Verification items for the finished model (mm, model axes). A direction names the side the tool comes from. Coordinates: 2 decimals unless noted, no trailing zeros. Order: outer loops, then holes, each group sorted by start corner. A loop starts at its lowest first (then second) coordinate and runs counter-clockwise, first axis right, second up.
Q1. Thickness scan on line 1 (X direction, y = 1.1, z = -20); line 2 (Z direction, x = -11, y = 2.15); line 3 (X direction, y = 2.5, z = 37.5). Record the ranges inside material, lowest first.
Q2. Cross-section at A-A, the plane x = -35. Record the boundary of the cut face in (y, z).
Q3. Set-up check for faces 5 (the flat face through (-60, 2, -38)), 6 (the flat face through (-30, 2, 25)), 7 (the cylindrical face through (-69, 3, -48)): record each of +Z, -Z, +X, -X, +Y, -Y from which the full face is reachable in a straight line by a thin tool's end or side.
Q4. Cross-section at B-B, the plane y = 3.35. Count the separate pieces of the cut face and the enclosed holes in it, and give its area (3 significant figures).
Q5. Draft check along Z on faces 1 (the cylindrical face through (-37, 2, -20)), 2 (the cylindrical face through (-33, 2, 20)), 3 (the flat face through (-70, 2, 1)), 4 (the cylindrical face through (-62, 3, -49)). Enter one of: pulls with the +Z half, pulls with the -Z half, needs draft (parallel to the pull), parting line crosses it, or undercut.
Q6. Depth check by flat-ended pin: P1, Ø1.5, axis at y = 3, z = -34.5, coming from the +X side; P2, Ø2.5, axis at x = -30.5, y = 3, coming from the +Z side; P3, Ø1.5, axis at x = -10.5, y = 3, coming from the -Z side. Enter the tip coordinate at first touch or a pass-through.
Q7. Cross-section at C-C, the plane z = 21. Record the boundary of the cut face in (x, y).
from build123d import *

# Parameters (mm, degrees)
SKETCH_2_R      = 2
EXTRUDE_1_DEPTH = 5
FILLET_1_R      = 5


with BuildPart() as part:
    # 스케치2 → 보스-돌출1 (new body)
    with BuildSketch(Plane(origin=(0, 0, 0), x_dir=(1, 0, 0), z_dir=(0, 1, 0))):
        Polygon((-60, -25), (-60, -50), (-70, -50), (-70, 50), (-60, 50), (-60, 25), (0, 25), (0, -25), align=None)
        with Locations(Location((-35, 20, 0), (0, 0, 270))):
            Circle(SKETCH_2_R, mode=Mode.SUBTRACT)
        with Locations(Location((-35, -20, 0), (0, 0, 90))):
            Circle(SKETCH_2_R, mode=Mode.SUBTRACT)
    extrude(amount=EXTRUDE_1_DEPTH)

    # 필렛1
    fillet_1_edges = [part.edges().sort_by_distance(p)[0] for p in [
        (-60, 2.5, -25),
        (0, 2.5, -25),
        (0, 2.5, 25),
        (-60, 2.5, 25),
        (-60, 2.5, 50),
        (-70, 2.5, 50),
        (-60, 2.5, -50),
        (-70, 2.5, -50),
    ]]
    fillet(fillet_1_edges, radius=FILLET_1_R - 0.0001)  # a hair under: the kernel refuses the full size


solid = part.part
Check values:
1. line 1: x = -70 to -37, -33 to 0
1. line 2: z = -25 to 25
1. line 3: x = -70 to -60
2. outline: (0, -25) - (5, -25) - (5, -22) - (0, -22) - close; (0, -18) - (5, -18) - (5, 18) - (0, 18) - close; (0, 22) - (5, 22) - (5, 25) - (0, 25) - close
3. face 5: -Z, +X, +Y, -Y
3. face 6: +Z, +X, +Y, -Y
3. face 7: -Z, -X, +Y, -Y
4. separate pieces: 1
4. enclosed holes: 2
4. area: 3,950 mm2
5. face 1: undercut
5. face 2: undercut
5. face 3: needs draft
5. face 4: pulls with the -Z half
6. P1: stops at x = -60
6. P2: stops at z = 25
6. P3: stops at z = -25
7. outline: (-70, 0) - (-36.73, 0) - (-36.73, 5) - (-70, 5) - close; (-33.27, 0) - (-0.1, 0) - (-0.1, 5) - (-33.27, 5) - close
